Geometry: final body of the model. Coordinates: model frame, mm. A direction names the side the tool comes from. Coordinates: 2 decimals unless noted, no trailing zeros. Write each loop counter-clockwise with the first axis right and the second up, starting at its lowest first coordinate (ties: lowest second). Pieces come first, ordered by that corner, then holes. Notation, with made-up numbers: (65, 18.25) -> (84, 18.25) arc R22 cw to (84, 40.25) -> close; hole circle Ø9 at (15.25, 39). An arc over 180 degrees is marked (long way). One line per item, written item: value.
```python
from build123d import *

# Parameters (mm, degrees)
SKETCH1_W                   = 58.547
SKETCH1_H                   = 44.577
SKETCH1_W_2                 = 47.625
SKETCH1_H_2                 = 26.797
BOSS_EXTRUDE1_DEPTH         = 5.715
BOSS_EXTRUDE2_REACH         = 57.19
SKETCH9_W                   = 1.5875
SKETCH9_H                   = 1.5875
FILLET11_R                  = 3.81
FILLET12_R                  = 3.81
F_1_4_CLEARANCE_HOLE1_D     = 6.7564
F_1_4_CLEARANCE_HOLE1_DEPTH = 8.89
F_1_4_CLEARANCE_HOLE1_TIP   = 2.029827343
F_6_32_TAPPED_HOLE1_D       = 2.7051
SKETCH22_W                  = 58.547
SKETCH22_H                  = 9.177220827
CUT_EXTRUDE4_DEPTH          = 41.791028073
FILLET14_R                  = 11.43
FILLET13_R                  = 11.43
SKETCH24_R                  = 1.5875
CUT_EXTRUDE5_DEPTH          = 11.43


with BuildPart() as part:
    # Sketch1 → Boss-Extrude1 (new, symmetric)
    with BuildSketch(Plane(origin=(0, 0, 0), x_dir=(0, 0, -1), z_dir=(1, 0, 0))):
        with Locations((2.921, 0)):
            Rectangle(SKETCH1_W, SKETCH1_H)
        Rectangle(SKETCH1_W_2, SKETCH1_H_2, mode=Mode.SUBTRACT)
    extrude(amount=BOSS_EXTRUDE1_DEPTH, both=True)

    # Sketch9 → Boss-Extrude2 (add, up to next)
    with BuildSketch(Plane.XY.offset(-23.8125), mode=Mode.PRIVATE) as boss_extrude2_sk1:
        with Locations((-4.92125, 12.60475)):
            Rectangle(SKETCH9_W, SKETCH9_H)
    boss_extrude2_tool1 = extrude(boss_extrude2_sk1.sketch, amount=BOSS_EXTRUDE2_REACH, mode=Mode.PRIVATE) - part.part
    # Sketch9 → Boss-Extrude2 (add, up to next)
    with BuildSketch(Plane.XY.offset(-23.8125), mode=Mode.PRIVATE) as boss_extrude2_sk2:
        with Locations((-4.92125, -12.60475)):
            Rectangle(SKETCH9_W, SKETCH9_H)
    boss_extrude2_tool2 = extrude(boss_extrude2_sk2.sketch, amount=BOSS_EXTRUDE2_REACH, mode=Mode.PRIVATE) - part.part
    add(boss_extrude2_tool1.solids().sort_by_distance((-4.92125, 12.60475, -23.8125))[0])
    add(boss_extrude2_tool2.solids().sort_by_distance((-4.92125, -12.60475, -23.8125))[0])

    # Fillet11
    fillet11_edges = [part.edges().sort_by_distance(p)[0] for p in [
        (-4.92125, -11.811, 23.8125),
        (-4.92125, -11.811, -23.8125),
        (-4.92125, 11.811, 23.8125),
        (-4.92125, 11.811, -23.8125),
    ]]
    fillet(fillet11_edges, radius=FILLET11_R)

    # Fillet12
    fillet12_edges = [part.edges().sort_by_distance(p)[0] for p in [
        (0.79375, 13.3985, 23.8125),
        (0.79375, -13.3985, 23.8125),
        (0.79375, -13.3985, -23.8125),
        (0.79375, 13.3985, -23.8125),
    ]]
    fillet(fillet12_edges, radius=FILLET12_R)

    # 1/4 Clearance Hole1
    with Locations(Plane(origin=(-2.530789808, 6.493019647, -32.1945), x_dir=(1, 0, 0), z_dir=(0, 0, -1))):
        with Locations((2.530789808, -0.936480353)):
            Hole(F_1_4_CLEARANCE_HOLE1_D / 2, depth=F_1_4_CLEARANCE_HOLE1_DEPTH)
            with Locations((0, 0, -(F_1_4_CLEARANCE_HOLE1_DEPTH + F_1_4_CLEARANCE_HOLE1_TIP / 2))):  # 118° drill point
                Cone(0, F_1_4_CLEARANCE_HOLE1_D / 2, F_1_4_CLEARANCE_HOLE1_TIP, mode=Mode.SUBTRACT)

    # #6-32 Tapped Hole1 (through all)
    with Locations(Plane(origin=(5.715, 17.955600219, 19.212274833), x_dir=(0, 0, 1), z_dir=(1, 0, 0))):
        with Locations((-27.657774833, 0.175600219), (-16.608774833, 0.175600219), (-5.559774833, 0.175600219), (-38.706774833, 0.175600219), (-38.706774833, 35.735600219), (-27.657774833, 35.735600219), (-16.608774833, 35.735600219), (-5.559774833, 35.735600219)):
            Hole(F_6_32_TAPPED_HOLE1_D / 2)

    # Sketch22 → Cut-Extrude4 (cut, through all)
    with BuildSketch(Plane.ZY.offset(5.715)):
        with Locations((-2.921, 25.353110414)):
            Rectangle(SKETCH22_W, SKETCH22_H)
    extrude(amount=-CUT_EXTRUDE4_DEPTH, mode=Mode.SUBTRACT)

    # Fillet14
    fillet14_edges = [part.edges().sort_by_distance(p)[0] for p in [
        (0, 20.7645, 26.3525),
        (0, -22.2885, 26.3525),
    ]]
    fillet(fillet14_edges, radius=FILLET14_R)

    # Fillet13
    # the kernel refuses this fillet: 11.43 mm, written as the material it takes off along each edge
    with BuildSketch(Plane(origin=(-34.29, 20.7645, -32.1945), x_dir=(0, 0, 1), z_dir=(1, 0, 0)), Plane(origin=(34.29, -22.2885, -32.1945), x_dir=(0, 0, 1), z_dir=(-1, 0, 0))) as fillet13_piece_1:
        with BuildLine():
            CenterArc((FILLET13_R, FILLET13_R), FILLET13_R, 180, 90)
            Line((0, FILLET13_R), (0, 0))
            Line((0, 0), (FILLET13_R, 0))
        make_face()
    extrude(amount=68.58, mode=Mode.SUBTRACT)

    # Sketch24 → Cut-Extrude5 (cut)
    with BuildSketch(Plane(origin=(5.715, 0, 0), x_dir=(0, 0, -1), z_dir=(1, 0, 0))):
        with Locations((19.4945, -17.78)):
            Circle(SKETCH24_R)
        with Locations((8.4455, -17.78)):
            Circle(SKETCH24_R)
        with Locations((-2.6035, -17.78)):
            Circle(SKETCH24_R)
        with Locations((-13.6525, -17.78)):
            Circle(SKETCH24_R)
        with Locations((-13.6525, 17.78)):
            Circle(SKETCH24_R)
        with Locations((-2.6035, 17.78)):
            Circle(SKETCH24_R)
        with Locations((8.4455, 17.78)):
            Circle(SKETCH24_R)
        with Locations((19.4945, 17.78)):
            Circle(SKETCH24_R)
    extrude(amount=-CUT_EXTRUDE5_DEPTH, mode=Mode.SUBTRACT)


solid = part.part
```
(1) Section C-C (y = 17.78). Return the cut outline in (x, z) (3 decimals), then the cut area to 3 significant figures.
Responses:
outline: (-5.715, -28.466) -> (5.715, -28.466) -> (5.715, -21.082) -> (-5.715, -21.082) -> close; (-5.715, -17.907) -> (5.715, -17.907) -> (5.715, -10.033) -> (-5.715, -10.033) -> close; (-5.715, -6.858) -> (5.715, -6.858) -> (5.715, 1.016) -> (-5.715, 1.016) -> close; (-5.715, 4.191) -> (5.715, 4.191) -> (5.715, 12.065) -> (-5.715, 12.065) -> close; (-5.715, 15.24) -> (5.715, 15.24) -> (5.715, 22.624) -> (-5.715, 22.624) -> close
area: 439 mm2
(2) Reachability of faces 4 (the flat face through (-5, -11.811, 0)), 5 (the cylindrical face through (0.72, 12.31, -22.67)), 6 (the flat face through (0, -22.288, -3)) from +Z, -Z, +X, -X, +Y, -Y: full face, straight path, thin tool, end or side. Return the list, or none.
Responses:
face 4: +X, -X
face 5: +X
face 6: +Z, -Z, +X, -X, -Y
(3) First-contact query: pin 1 (2.5 mm diameter, centred on y = -17.78, z = -19.49, fed in from -X); pin 2 (5 mm diameter, centred on x = 1, y = -16.5, fed in from -Z). Flat tips, straight axial feed; report the tip coordinate or a pass-through.
Responses:
pin 1: passes through
pin 2: stops at z = -31.75
(4) Section B-B (x = 4). State how many separate pieces and enclosed holes the cut face has, then the cut area to 3 significant figures.
Responses:
separate pieces: 1
enclosed holes: 9
area: 1,080 mm2
(5) Pull-direction query (Z, two-part tool) for faces 1 (the cylindrical face through (0.08, -18.851, -28.935)), 2 (the flat face through (-5.715, -15, -10)), 3 (the flat face through (1, -13.398, 0)); classes: released by +Z, released by -Z, zero draft, split by the parting line, or undercut.
Responses:
face 1: released by -Z
face 2: zero draft
face 3: undercut
(6) Line query: line 1 (Y direction, x = -2.25, z = -8.5); line 2 (Y direction, x = -1.5, z = -15); line 3 (Z direction, x = -2.25, y = -16.5). Output: solid intervals per line, ascending. Write a range as [from, to].
Responses:
line 1: y = [-22.29, -19.37], [-16.19, -13.4], [13.4, 16.19], [19.37, 20.76]
line 2: y = [-22.29, -13.4], [13.4, 20.76]
line 3: z = [-30.71, -20.43], [-18.56, -9.38], [-7.51, 1.66], [3.54, 12.71], [14.59, 24.86]
(7) Section A-A (y = -3.5). Return the cut outline in (x, z) (1 decimal).
Responses:
outline: (-5.7, -32.2) -> (5.7, -32.2) -> (5.7, -23.8) -> (-5.7, -23.8) -> close; (-5.7, 23.8) -> (5.7, 23.8) -> (5.7, 26.4) -> (-5.7, 26.4) -> close
